```python
from build123d import *

# Parameters (mm, degrees)
F0_W           = 304.8
F0_H           = 203.2
F1_DEPTH       = 25.4
F3_SIZE        = 50.8
F4_W           = 228.6
F4_H           = 25.4
F5_DEPTH       = 25.4
F6_R           = 6.35
F8_D           = 9.525
F8_CBORE_D     = 12.7
F8_CBORE_DEPTH = 12.7
F10_D          = 6.35
F12_D          = 12.7
F12_DEPTH      = 12.7
F12_TIP        = 3.8154649308


with BuildPart() as f1:
    # F0 (on Top) → F1 (new body)
    with BuildSketch(Plane.XY):
        with Locations((0.9524989873, 1.4589339421)):
            Rectangle(F0_W, F0_H)
    extrude(amount=F1_DEPTH)

    # F3
    f3_edges = [f1.edges().sort_by_distance(p)[0] for p in [
        (-151.447501, 103.058934, 12.7),
        (153.352499, 103.058934, 12.7),
    ]]
    chamfer(f3_edges, length=F3_SIZE)

    # F4 (on face) → F5 (cut)
    with BuildSketch(Plane.XZ.offset(100.1410660579)):
        with Locations((0.9524989873, 12.7)):
            Rectangle(F4_W, F4_H)
    extrude(amount=-F5_DEPTH, mode=Mode.SUBTRACT)

    # F6
    f6_edges = [f1.edges().sort_by_distance(p)[0] for p in [
        (-113.347501, -100.141066, 12.7),
        (-113.347501, -74.741066, 12.7),
        (115.252499, -74.741066, 12.7),
        (115.252499, -100.141066, 12.7),
        (153.352499, -100.141066, 12.7),
        (-151.447501, -100.141066, 12.7),
    ]]
    fillet(f6_edges, radius=F6_R)

    # F8 (through all)
    with Locations(Plane.XY.offset(25.4)):
        with Locations((-132.3975010127, -81.0910660579), (-132.3975010127, -4.8910660579), (134.3024989873, -4.8910660579), (134.3024989873, -81.0910660579)):
            CounterBoreHole(F8_D / 2, F8_CBORE_D / 2, F8_CBORE_DEPTH)

    # F10 (through all)
    with Locations(Plane.XY.offset(25.4)):
        with Locations((13.6524989873, -62.0410660579), (77.1524989873, -62.0410660579)):
            Hole(F10_D / 2)

    # F12
    with Locations(Plane.XY.offset(25.4)):
        with Locations((-126.0475010127, 34.0471339421), (127.9524989873, 34.0471339421)):
            Hole(F12_D / 2, depth=F12_DEPTH)
            with Locations((0, 0, -(F12_DEPTH + F12_TIP / 2))):  # 118° drill point
                Cone(0, F12_D / 2, F12_TIP, mode=Mode.SUBTRACT)


solid = f1.part
```
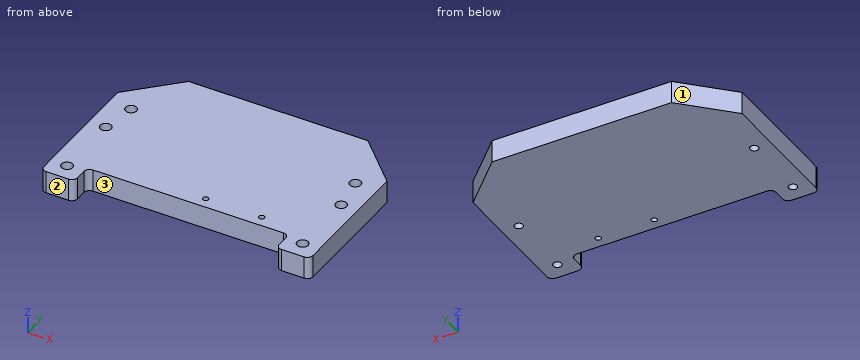
The model under review builds one solid part; all positions refer to its coordinate system, in mm. Face numbers are marked on the shaded views. Coordinates: 2 decimals unless noted, no trailing zeros. Order: outer loops, then holes, each group sorted by start corner. A loop starts at its lowest first (then second) coordinate and runs counter-clockwise, first axis right, second up. Notation, with made-up numbers: M 62.25,89.5 L 81.25,89.5 A32 cw 81.25,115.5 Z; hole C 52.5,-32.75 d8. An arc over 180 degrees is marked long. One line per question, with ' | ' between items.
(1) Add section B-B, the plane x = -29. Write out the cut boundary in (y, z).
Geometry results:
outline: M -74.74,0 L 103.06,0 L 103.06,25.4 L -74.74,25.4 Z
(2) The part is to be moulded in two halves that separate along X. For the marked faces 1, 2 and 3, say which applies: +X half, -X half, draft (parallel to the pull), parting line (faces both ways), or undercut.
Geometry results:
face 1: -X half | face 2: draft | face 3: undercut
(3) Add section A-A, the plane z = 5.25. State how many separate pieces and enclosed holes the cut face has, then the cut area to 3 significant figures.
Geometry results:
separate pieces: 1 | enclosed holes: 6 | area: 53,200 mm²
(4) Add section C-C, the plane y = 81.5. Write out the cut boundary in (x, z), then the cut area to 3 significant figures.
Geometry results:
outline: M -122.21,0 L 124.11,0 L 124.11,25.4 L -122.21,25.4 Z | area: 6,260 mm²
(5) Insertion check: pin 1 (11 mm diameter, centred on x = -132.4, y = -81.09, fed in from +Z); pin 2 (5.5 mm diameter, centred on x = 77.15, y = -62.04, fed in from -Z); pin 3 (3 mm diameter, centred on x = -105.5, z = 21, fed in from -Y). Each pin has a flat end and moves straight along its axis. Give the tip position at first contact, or say it passes through.
Geometry results:
pin 1: stops at z = 12.7 | pin 2: passes through | pin 3: stops at y = -74.74
(6) For probe 1 along X at (y, z) = (-85.5, 3.25); probe 2 along X at (y, z) = (-2, 8.75); probe 3 along X at (y, z) = (-61, 14.25), list the stretches that pass through material, from the lowest coordinate up. Write a range as from..to.
Geometry results:
probe 1: x = -151.45..-134.2, -130.6..-113.35, 115.25..132.5, 136.1..153.35 | probe 2: x = -151.45..-136.18, -128.61..130.52, 138.09..153.35 | probe 3: x = -151.45..10.65, 16.65..74.15, 80.15..153.35
